The listing builds one solid part. Answer for the finished solid, in the listing's coordinates (mm). A direction names the side the tool comes from. Give positions to 0.01 mm unless a question says otherwise; leave off trailing zeros. Write each loop counter-clockwise with the first axis right and the second up, starting at its lowest first coordinate (ties: lowest second). Pieces come first, ordered by that corner, then holes. Notation, with made-up numbers: (9, -32.75) - (45, -32.75) arc R6 ccw to (45, -26.75) - close; hole circle Ø4 at (2, -26.75). An arc over 180 degrees is marked (long way). Use a Markdown table: item, result. Add a question column.
from build123d import *

# Parameters (mm, degrees)
ESBO_O2_R                         = 4
ESBO_O2_R_2                       = 4.25
ESBO_O2_R_3                       = 11
RESSALTO_EXTRUS_O1_DEPTH          = 20
RESSALTO_EXTRUS_O2_DEPTH          = 10
FILETE1_R                         = 3
CORTE_EXTRUS_O1_DEPTH             = 10
REBAIXO_PARA_SHCS_M61_D           = 6.6
REBAIXO_PARA_SHCS_M61_CBORE_D     = 11
REBAIXO_PARA_SHCS_M61_CBORE_DEPTH = 6


with BuildPart() as part:
    # Esboço2 → Ressalto-extrusão1 (new body)
    with BuildSketch(Plane.XY):
        with BuildLine():
            Line((250, 102.212171493), (250, 76.212189341))
            ThreePointArc((250, 76.212189341), (248.828427125, 73.383762216), (246, 72.212189341))
            Line((246, 72.212189341), (194, 72.212189341))
            ThreePointArc((194, 72.212189341), (191.171572875, 73.383762216), (190, 76.212189341))
            Line((190, 76.212189341), (190, 102.212171493))
            Line((190, 102.212171493), (190, 135.998985905))
            ThreePointArc((190, 135.998985905), (191.141807012, 141.73923739), (194.393398282, 146.605587623))
            Line((194.393398282, 146.605587623), (209.393398282, 161.605587623))
            ThreePointArc((209.393398282, 161.605587623), (220, 165.998985905), (230.606601718, 161.605587623))
            Line((230.606601718, 161.605587623), (245.606601718, 146.605587623))
            ThreePointArc((245.606601718, 146.605587623), (248.858192988, 141.73923739), (250, 135.998985905))
            Line((250, 135.998985905), (250, 102.212171493))
        make_face()
        with Locations((198, 112.212189341)):
            Circle(ESBO_O2_R, mode=Mode.SUBTRACT)
        with Locations((242, 112.212189341)):
            Circle(ESBO_O2_R_2, mode=Mode.SUBTRACT)
        with Locations((220, 143.362189341)):
            Circle(ESBO_O2_R_3, mode=Mode.SUBTRACT)
    extrude(amount=RESSALTO_EXTRUS_O1_DEPTH)

    # Esboço3 → Ressalto-extrusão2 (add)
    with BuildSketch(Plane(origin=(0, 0, 0), x_dir=(-1, 0, 0), z_dir=(0, 0, -1))):
        with BuildLine():
            Line((-250, 111.697903626), (-250, 102.212171493))
            Line((-250, 102.212171493), (-190, 102.212171493))
            Line((-190, 102.212171493), (-190, 111.697903626))
            Line((-190, 111.697903626), (-194.033198996, 111.697903626))
            ThreePointArc((-194.033198996, 111.697903626), (-198, 108.212189341), (-201.966801004, 111.697903626))
            Line((-201.966801004, 111.697903626), (-237.781231198, 111.697903626))
            ThreePointArc((-237.781231198, 111.697903626), (-242, 107.962189341), (-246.218768802, 111.697903626))
            Line((-246.218768802, 111.697903626), (-250, 111.697903626))
        make_face()
    extrude(amount=RESSALTO_EXTRUS_O2_DEPTH)

    # Filete1
    filete1_edges = [part.edges().sort_by_distance(p)[0] for p in [
        (219.874016101, 111.697903626, -10),
        (248.109384401, 111.697903626, -10),
        (250, 106.955037559, -10),
        (190, 106.955037559, -10),
        (192.016599498, 111.697903626, -10),
    ]]
    fillet(filete1_edges, radius=FILETE1_R)

    # Esboço4 → Corte-extrusão1 (cut)
    with BuildSketch(Plane(origin=(0, 0, 0), x_dir=(-1, 0, 0), z_dir=(0, 0, -1))):
        with BuildLine():
            Line((-194.033198996, 111.697903626), (-190, 111.697903626))
            Line((-190, 111.697903626), (-190, 135.998985905))
            ThreePointArc((-190, 135.998985905), (-191.141807012, 141.73923739), (-194.393398282, 146.605587623))
            Line((-194.393398282, 146.605587623), (-209.393398282, 161.605587623))
            ThreePointArc((-209.393398282, 161.605587623), (-220, 165.998985905), (-230.606601718, 161.605587623))
            Line((-230.606601718, 161.605587623), (-245.606601718, 146.605587623))
            ThreePointArc((-245.606601718, 146.605587623), (-248.858192988, 141.73923739), (-250, 135.998985905))
            Line((-250, 135.998985905), (-250, 111.697903626))
            Line((-250, 111.697903626), (-246.218768802, 111.697903626))
            ThreePointArc((-246.218768802, 111.697903626), (-242, 116.462189341), (-237.781231198, 111.697903626))
            Line((-237.781231198, 111.697903626), (-201.966801004, 111.697903626))
            ThreePointArc((-201.966801004, 111.697903626), (-198, 116.212189341), (-194.033198996, 111.697903626))
        make_face()
    extrude(amount=-CORTE_EXTRUS_O1_DEPTH, mode=Mode.SUBTRACT)

    # Rebaixo para SHCS M61 (through all)
    with Locations(Plane.XY.offset(20)):
        with Locations((235, 87.212189341), (205, 87.212189341)):
            CounterBoreHole(REBAIXO_PARA_SHCS_M61_D / 2, REBAIXO_PARA_SHCS_M61_CBORE_D / 2, REBAIXO_PARA_SHCS_M61_CBORE_DEPTH)


solid = part.part
1. For a pull along Y with two mould halves and no side action, classify faces 1 (the cylindrical face through (220.04, 110.84, -9.1)), 2 (the flat face through (190, 99, 9)), 3 (the cylindrical face through (234.284, 92.665, 17.042)), 4 (the flat face through (239, 87, 14)) as released by +Y, released by -Y, zero draft, split by the parting line, or undercut.
2. Given P1, Ø14.5, axis at x = 235, y = 87.21, coming from the -Z side; P2, Ø5.5, axis at x = 205, y = 87.21, coming from the +Z side; P3, Ø16.5, axis at x = 234.5, y = 150, coming from the -Z side; P4, Ø4, axis at y = 149.5, z = 10, coming from the +X side, each flat-ended and moving along its own axis, determine where each tip first touches the part or whether it passes through.
3. The part is cut by section C-C (z = 1.5). Give the vertices of the cut face in (x, y), and give its area (3 significant figures).
4. The part is cut by section D-D (z = -4.5). Give the vertices of the cut face in (x, y), and give its area (3 significant figures).
5. The part is cut by section B-B (y = 110). Give the vertices of the cut face in (x, z).
6. Consider L1, parallel to X at y = 89.5, z = 10; L2, parallel to Y at x = 205, z = 9; L3, parallel to Z at x = 220.5, y = 93.5. Determine where each line is inside the solid, lowest interval first. Write a range as [from, to].
7. The part is cut by section A-A (x = 220). Give the vertices of the cut face in (y, z), and give its area (3 significant figures).
8. Which of the six approach directions +Z, -Z, +X, -X, +Y, -Y give full straight-line access (tool end or side, diameter ignored) to faces 5 (the cylindrical face through (249.14, 106.89, -9.1)), 6 (the flat face through (192, 111.698, 1)), 7 (the flat face through (220, 87, 0)), 8 (the flat face through (204.9, 83.6, 14))?
Check values:
| question | item | result |
|---|---|---|
| 1 | face 1 | released by +Y |
| 1 | face 2 | zero draft |
| 1 | face 3 | undercut |
| 1 | face 4 | undercut |
| 2 | P1 | stops at z = 0 |
| 2 | P2 | passes through |
| 2 | P3 | stops at z = 10 |
| 2 | P4 | stops at x = 244.71 |
| 3 | outline | (190, 76.21) arc R4 ccw to (194, 72.21) - (246, 72.21) arc R4 ccw to (250, 76.21) - (250, 111.7) - (246.22, 111.7) arc R4.25 cw to (237.78, 111.7) - (201.97, 111.7) arc R4 cw to (194.03, 111.7) - (190, 111.7) - close; hole circle Ø6.6 at (205, 87.21); hole circle Ø6.6 at (235, 87.21) |
| 3 | area | 2,250 mm2 |
| 4 | outline | (190, 102.21) - (250, 102.21) - (250, 111.7) - (246.22, 111.7) arc R4.25 cw to (237.78, 111.7) - (201.97, 111.7) arc R4 cw to (194.03, 111.7) - (190, 111.7) - close |
| 4 | area | 524 mm2 |
| 5 | outline | (190, -7) arc R3 ccw to (191.7, -9.7) - (194.67, -9.7) - (194.67, 20) - (190, 20) - close; (201.33, -9.7) - (238.37, -9.7) - (238.37, 20) - (201.33, 20) - close; (245.63, -9.7) - (248.3, -9.7) arc R3 ccw to (250, -7) - (250, 20) - (245.63, 20) - close |
| 6 | L1 | x = [190, 202.62], [207.38, 232.62], [237.38, 250] |
| 6 | L2 | y = [72.21, 83.91], [90.51, 111.7] |
| 6 | L3 | z = [0, 20] |
| 7 | outline | (72.21, 0) - (102.21, 0) - (102.21, -10) - (108.7, -10) arc R3 ccw to (111.7, -7) - (111.7, 10) - (132.36, 10) - (132.36, 20) - (72.21, 20) - close; (154.36, 10) - (166, 10) - (166, 20) - (154.36, 20) - close |
| 7 | area | 1,210 mm2 |
| 8 | face 5 | -Z, +X, +Y, -Y |
| 8 | face 6 | -Z, +X, -X, +Y |
| 8 | face 7 | -Z, +X, -X, -Y |
| 8 | face 8 | +Z |
